For this review, use the dimensioned drawing (mm, ordinates from the lowest corner) and the shaded views. A direction names the side the tool comes from. Give positions to 0.01 mm unless a question says otherwise; leave off trailing zeros. Loops run counter-clockwise (first coordinate to the right, second up) from the corner with the lowest first, then second, coordinate; pieces in that order, holes last. Notation, with made-up numbers: M 14.25,3.25 L 25.25,3.25 A31 ccw 25.25,37.25 Z; hole C -7,-32 d7. An arc over 180 degrees is marked long. Use CSV: the item, a comma, the result in double quotes. Start each with the question number.
1. To check wall thickness, follow line 1 (X direction, y = 8.75, z = 1.9); line 2 (Y direction, x = 14, z = 2.9); line 3 (X direction, y = 16.5, z = 1.95). State the ranges of each line that lie inside material, in increasing order. Write a range as [from, to].
2. Take a section at A-A, the plane x = 6.25. Write out the cut boundary in (y, z), and give its area (3 significant figures).
3. Tool access review of the marked faces 1, 2, 3 and 4: name each direction out of +Z, -Z, +X, -X, +Y, -Y from which nothing blocks a thin tool from reaching the whole face with its end or side.
4. Take a section at C-C, the plane x = 17.5. Write out the cut boundary in (y, z).
5. Take a section at D-D, the plane x = 26. Write out the cut boundary in (y, z), and give its area (3 significant figures).
6. Insertion check: P1, Ø1, axis at x = 21, y = 4, coming from the +Z side; P2, Ø1, axis at y = 10.5, z = 3, coming from the -X side; P3, Ø1.4, axis at x = 5, z = 3, coming from the +Y side. Each pin has a flat end and moves straight along its axis. Give the tip position at first contact, or say it passes through.
7. Take a section at B-B, the plane y = 11.75. Write out the cut boundary in (x, z), and give its area (3 significant figures).
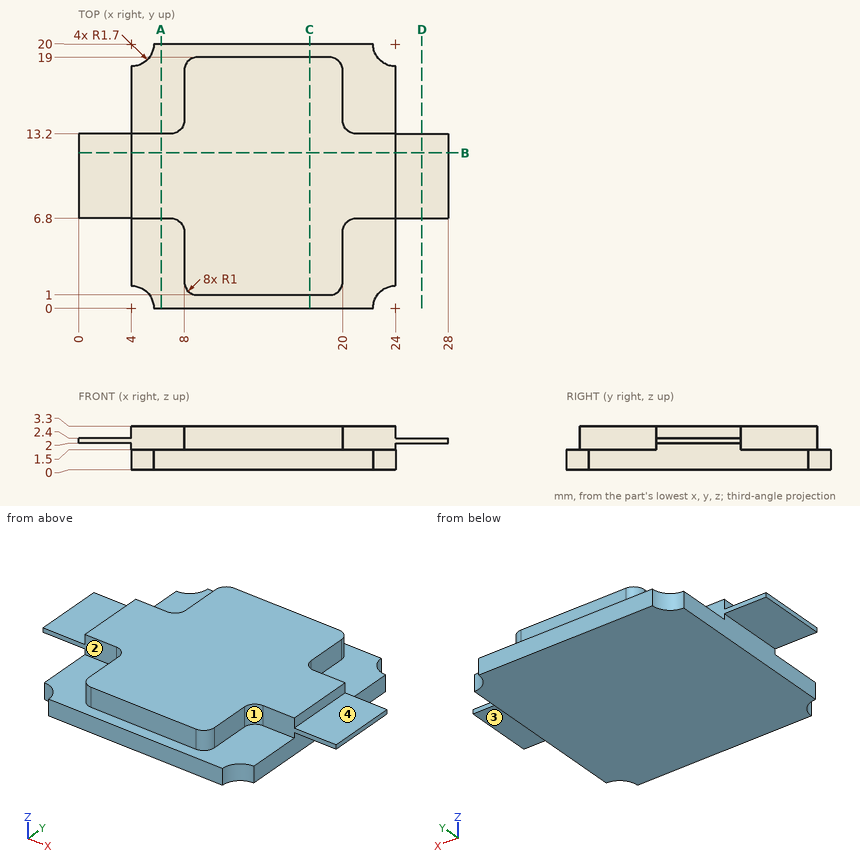
Result set:
1,line 1,"[4, 24]"
1,line 2,"[1, 19]"
1,line 3,"[8, 20]"
2,outline,"M 0,0 L 20,0 L 20,1.5 L 13.2,1.5 L 13.2,3.3 L 6.8,3.3 L 6.8,1.5 L 0,1.5 Z"
2,area,"41.5 mm2"
3,face 1,"+Z, +X, -Y"
3,face 2,"+Z, -X, -Y"
3,face 3,"-Z, +X, +Y, -Y"
3,face 4,"+Z, +X, +Y, -Y"
4,outline,"M 0,0 L 20,0 L 20,1.5 L 19,1.5 L 19,3.3 L 1,3.3 L 1,1.5 L 0,1.5 Z"
5,outline,"M 6.8,2 L 13.2,2 L 13.2,2.4 L 6.8,2.4 Z"
5,area,"2.56 mm2"
6,P1,"z = 1.5"
6,P2,"x = 4"
6,P3,"y = 13.2"
7,outline,"M 0,2 L 4,2 L 4,0 L 24,0 L 24,2 L 28,2 L 28,2.4 L 24,2.4 L 24,3.3 L 4,3.3 L 4,2.4 L 0,2.4 Z"
7,area,"69.2 mm2"
